Read the model definition and answer for the solid it produces. Units are mm, in the model's axes. A direction names the side the tool comes from. Coordinates: 2 decimals unless noted, no trailing zeros. Order: outer loops, then holes, each group sorted by start corner. A loop starts at its lowest first (then second) coordinate and runs counter-clockwise, first axis right, second up. Notation, with made-up numbers: (74.5, 25.25) -> (90.5, 25.25) arc R8 cw to (90.5, 33.25) -> close; hole circle Ø6 at (11.25, 84.25). An arc over 180 degrees is marked (long way). Answer as a JSON object with one key per item and string values. Group by question number.
1) Section C-C on z = 2 is taken. Determine the outline of the cut face in (x, y), and give its area (3 significant figures).
2) A tool of negligible diameter and unlimited length cuts with its end or side. For faces 4 (the cylindrical face through (3.9, 3.7, 3.9)), 5 (the flat face through (3, 0, 8)), from which of +Z, -Z, +X, -X, +Y, -Y can it reach the whole face along a straight path? Write none if from no direction.
3) Determine the mould class of faces 1 (the cylindrical face through (-3.811, -3.833, 3.944)), 2 (the flat face through (1.1, 1.1, -3)), 3 (the cylindrical face through (-0.54, 2.44, -1.48)) for opening direction X: released by +X, released by -X, zero draft, split by the parting line, or undercut.
4) Given pin 1 (3 mm diameter, centred on y = -7, z = 6.5, fed in from -X); pin 2 (1 mm diameter, centred on x = 11.5, y = 4, fed in from -Z); pin 3 (5 mm diameter, centred on y = -8, z = -1.5, fed in from +X); pin 4 (3 mm diameter, centred on x = 0, y = 0, fed in from +Z), each flat-ended and moving along its own axis, determine where each tip first touches the part or whether it passes through.
5) Section D-D on z = -0.5 is taken. Determine the outline of the cut face in (x, y), and give its area (3 significant figures).
6) Section A-A on x = 0 is taken. Determine the outline of the cut face in (y, z), and give its area (3 significant figures).
7) Consider L1, parallel to Y at x = 0, z = 1.5; L2, parallel to X at y = 0, z = -0.5; L3, parallel to X at y = 7, z = 3.25. Determine where each line is inside the solid, lowest interval first.
from build123d import *

# Parameters (mm, degrees)
F0_R     = 15
F0_R_2   = 1.4
F1_DEPTH = 8
F2_R     = 1.5
F3_R     = 1.5
F4_R     = 2.5
F5_DEPTH = 3
F6_R     = 1.4
F7_DEPTH = 25


with BuildPart() as f1:
    # F0 (on Top) → F1 (new body)
    with BuildSketch(Plane.XY):
        Circle(F0_R)
        with BuildLine():
            ThreePointArc((-9.796631, -2.006496), (-3.744207, -3.896689), (-1.614051, -9.868882))
            ThreePointArc((-1.614051, -9.868882), (-6.928578, -7.210743), (-9.796631, -2.006496))
        make_face(mode=Mode.SUBTRACT)
        with BuildLine():
            ThreePointArc((1.531464, -9.882035), (3.685338, -3.80578), (9.827695, -1.848356))
            ThreePointArc((9.827695, -1.848356), (6.956481, -7.183827), (1.531464, -9.882035))
        make_face(mode=Mode.SUBTRACT)
        with BuildLine():
            ThreePointArc((-9.80076, 1.986231), (-6.865646, 7.270688), (-1.421798, 9.898408))
            ThreePointArc((-1.421798, 9.898408), (-3.712984, 3.932034), (-9.80076, 1.986231))
        make_face(mode=Mode.SUBTRACT)
        Circle(F0_R_2, mode=Mode.SUBTRACT)
        with BuildLine():
            ThreePointArc((9.855809, 1.692051), (3.799696, 3.798731), (1.694555, 9.855378))
            ThreePointArc((1.694555, 9.855378), (7.071966, 7.070169), (9.855809, 1.692051))
        make_face(mode=Mode.SUBTRACT)
    extrude(amount=F1_DEPTH)

    # F2
    f2_edges = [f1.edges().sort_by_distance(p)[0] for p in [
        (-15, 0, 8),
    ]]
    fillet(f2_edges, radius=F2_R)

    # F3
    f3_edges = [f1.edges().sort_by_distance(p)[0] for p in [
        (-15, 0, 0),
    ]]
    fillet(f3_edges, radius=F3_R)

    # F4 (on face) → F5 (join)
    with BuildSketch(Plane(origin=(0, 0, 0), x_dir=(1, 0, 0), z_dir=(0, 0, -1))):
        Circle(F4_R)
    extrude(amount=F5_DEPTH)

    # F6 (on face) → F7 (cut)
    with BuildSketch(Plane(origin=(0, 0, -3), x_dir=(1, 0, 0), z_dir=(0, 0, -1))):
        Circle(F6_R)
    extrude(amount=-F7_DEPTH, mode=Mode.SUBTRACT)


solid = f1.part
Worked answers:
{
 "1": {"outline": "circle Ø30 at (0, 0); hole (-9.8, -2.01) arc R10 ccw to (-1.61, -9.87) arc R7.1 ccw to start; hole (-9.8, 1.99) arc R7.39 ccw to (-1.42, 9.9) arc R10 ccw to start; hole circle Ø2.8 at (0, 0); hole (1.53, -9.88) arc R10 ccw to (9.83, -1.85) arc R7.25 ccw to start; hole (1.69, 9.86) arc R7.36 ccw to (9.86, 1.69) arc R10 ccw to start", "area": "554 mm²"},
 "2": {"face 4": "+Z, -Z", "face 5": "+Z, +X, -X, +Y, -Y"},
 "3": {"face 1": "undercut", "face 2": "zero draft", "face 3": "split by the parting line"},
 "4": {"pin 1": "stops at x = -13.96", "pin 2": "stops at z = 0", "pin 3": "stops at x = 13.11", "pin 4": "stops at z = 8"},
 "5": {"outline": "circle Ø5 at (0, 0); hole circle Ø2.8 at (0, 0)", "area": "13.5 mm²"},
 "6": {"outline": "(-15, 1.5) arc R1.5 ccw to (-13.5, 0) -> (-2.5, 0) -> (-2.5, -3) -> (-1.4, -3) -> (-1.4, 8) -> (-13.5, 8) arc R1.5 ccw to (-15, 6.5) -> close; (1.4, -3) -> (2.5, -3) -> (2.5, 0) -> (13.5, 0) arc R1.5 ccw to (15, 1.5) -> (15, 6.5) arc R1.5 ccw to (13.5, 8) -> (1.4, 8) -> close", "area": "222 mm²"},
 "7": {"L1": "y = -15 to -1.4, 1.4 to 15", "L2": "x = -2.5 to -1.4, 1.4 to 2.5", "L3": "x = -13.27 to -7.14, -1.77 to 1.92, 7.14 to 13.27"}
}
